```python
from build123d import *

# Parameters (mm, degrees)
SKETCH1_W               = 96
SKETCH1_H               = 64
BOSS_EXTRUDE1_DEPTH     = 20
BOSS_EXTRUDE2_DEPTH     = 32
BOSS_EXTRUDE3_DEPTH     = 12
SKETCH8_R               = 26
SKETCH8_R_2             = 16
BOSS_EXTRUDE4_DEPTH     = 32
CUT_EXTRUDE1_DEPTH      = 177.853582377
CUT_EXTRUDE1_DEPTH_BACK = 177.853582377
SKETCH9_R               = 16
RIB9_START              = -6
RIB9_DEPTH              = 12
FILLET1_R               = 1


with BuildPart() as part:
    # Sketch1 → Boss-Extrude1 (new body)
    with BuildSketch(Plane(origin=(0, 0, 0), x_dir=(1, 0, 0), z_dir=(0, 1, 0))):
        Rectangle(SKETCH1_W, SKETCH1_H)
    extrude(amount=-BOSS_EXTRUDE1_DEPTH)

    # Sketch4 → Boss-Extrude2 (add, symmetric)
    with BuildSketch(Plane(origin=(0, 0, 0), x_dir=(0, 0, -1), z_dir=(1, 0, 0))):
        with BuildLine():
            Line((20, -20), (32, -20))
            Line((32, -20), (32, 44.558859159))
            ThreePointArc((32, 44.558859159), (32.694245739, 49.069446152), (34.712719336, 53.162505705))
            Line((34.712719336, 53.162505705), (68.042689949, 100.762636801))
            Line((68.042689949, 100.762636801), (58.212865417, 107.645554037))
            Line((58.212865417, 107.645554037), (22.712719336, 56.946091171))
            ThreePointArc((22.712719336, 56.946091171), (20.694245739, 52.853031619), (20, 48.342444626))
            Line((20, 48.342444626), (20, -20))
        make_face()
    extrude(amount=BOSS_EXTRUDE2_DEPTH, both=True)

    # Sketch6 → Boss-Extrude3 (add)
    with BuildSketch(Plane(origin=(0, 8.063203075, 11.515447399), x_dir=(1, 0, 0), z_dir=(0, 0.573576436351053, 0.819152044288987))):
        with BuildLine():
            Line((-32, 121.567603544), (32, 121.567603544))
            ThreePointArc((32, 121.567603544), (0, 153.567603544), (-32, 121.567603544))
        make_face()
    extrude(amount=-BOSS_EXTRUDE3_DEPTH)

    # Sketch8 → Boss-Extrude4 (add)
    with BuildSketch(Plane(origin=(0, 8.063203075, 11.515447399), x_dir=(1, 0, 0), z_dir=(0, 0.573576436351053, 0.819152044288987))):
        with Locations(Location((0, 121.567603544, 0), (0, 0, 270))):
            Circle(SKETCH8_R)
        with Locations(Location((0, 121.567603544, 0), (0, 0, 270))):
            Circle(SKETCH8_R_2, mode=Mode.SUBTRACT)
    extrude(amount=BOSS_EXTRUDE4_DEPTH)

    # Sketch9 → Cut-Extrude1 (cut, two sides: drawn at the far end of the back side and taken through both)
    with BuildSketch(Plane(origin=(0, 8.063203075, 11.515447399), x_dir=(1, 0, 0), z_dir=(0, 0.573576436351053, 0.819152044288987)).offset(-CUT_EXTRUDE1_DEPTH_BACK)):
        with Locations(Location((0, 121.567603544, 0), (0, 0, 270))):
            Circle(SKETCH9_R)
    extrude(amount=CUT_EXTRUDE1_DEPTH + CUT_EXTRUDE1_DEPTH_BACK, mode=Mode.SUBTRACT)

    # Rib9: read off the stored shape, not the designer's step
    # Rib9 outline → Rib9 (add)
    with BuildSketch(Plane(origin=(0, 0, 0), x_dir=(0, 0, -1), z_dir=(1, 0, 0)).offset(RIB9_START)):
        with BuildLine():
            Line((22.712719336, 56.946091171), (43.702401809, 86.922464357))
            Line((43.702401809, 86.922464357), (22.404448657, 101.835451702))
            Line((22.404448657, 101.835451702), (1.414766184, 71.859078516))
            ThreePointArc((1.414766184, 71.859078516), (-4.102394981, 60.671382406), (-6, 48.342444626))
            ThreePointArc((-6, 48.342444626), (-12.91230776, 20.897080936), (-32, 0))
            Line((-32, 0), (20, 0))
            Line((20, 0), (20, 48.342444626))
            ThreePointArc((20, 48.342444626), (20.694245739, 52.853031619), (22.712719336, 56.946091171))
        make_face()
    extrude(amount=RIB9_DEPTH)

    # Fillet1
    # the kernel refuses this fillet: 1 mm, written as the material it adds along each edge
    with BuildSketch(Plane(origin=(-7, 1, -19), x_dir=(1, 0, 0), z_dir=(0, -1, 0))) as fillet1_piece_1_section:
        Polygon((0, 0), (FILLET1_R * 1.02, 0), (FILLET1_R * 1.02, -FILLET1_R * 1.02), (0, -FILLET1_R * 1.02), align=None)
    fillet1_piece_1 = extrude(amount=FILLET1_R * 1.02, mode=Mode.PRIVATE)
    fillet1_piece_1 = fillet1_piece_1 - Plane(origin=(-7, 1, -19), x_dir=(-0.7071067811865475, 0, 0.7071067811865475), z_dir=(0, -1, 0)) * Sphere(FILLET1_R, mode=Mode.PRIVATE)
    add(fillet1_piece_1)
    with BuildSketch(Plane(origin=(7, 1, -19), x_dir=(0, 0, -1), z_dir=(-1, 0, 0))) as fillet1_piece_2_section:
        Polygon((0, 0), (FILLET1_R * 1.02, 0), (FILLET1_R * 1.02, FILLET1_R * 1.02), (0, FILLET1_R * 1.02), align=None)
    fillet1_piece_2 = extrude(amount=FILLET1_R * 1.02, mode=Mode.PRIVATE)
    fillet1_piece_2 = fillet1_piece_2 - Plane(origin=(7, 1, -19), x_dir=(0, 0.7071067811865475, 0.7071067811865476), z_dir=(-1, 0, 0)) * Sphere(FILLET1_R, mode=Mode.PRIVATE)
    add(fillet1_piece_2)
    with BuildSketch(Plane(origin=(-6, 0, 34.5), x_dir=(-1, 0, 0), z_dir=(0, 0, -1))) as fillet1_piece_3_section:
        with BuildLine():
            CenterArc((FILLET1_R, FILLET1_R), FILLET1_R, 180, 90)
            Line((0, FILLET1_R), (0, 0))
            Line((0, 0), (FILLET1_R, 0))
        make_face()
    fillet1_piece_3 = extrude(amount=53.5, mode=Mode.PRIVATE)
    fillet1_piece_3 = fillet1_piece_3 - Plane(origin=(-6, 48.342444627, 63.942152933), x_dir=(0, -1.6764948068756696e-11, -1.0), z_dir=(-1, 0, 0)) * Cylinder(57.942152933, 111, mode=Mode.PRIVATE)
    add(fillet1_piece_3)
    with BuildSketch(Plane(origin=(-6, 1, -20), x_dir=(0, 0, 1), z_dir=(0, 1, 0)), Plane(origin=(6, 1, -20), x_dir=(1, 0, 0), z_dir=(0, 1, 0))) as fillet1_piece_4:
        with BuildLine():
            CenterArc((FILLET1_R, -FILLET1_R), FILLET1_R, 90, 90)
            Line((0, -FILLET1_R), (0, 0))
            Line((0, 0), (FILLET1_R, 0))
        make_face()
    extrude(amount=47.342444626)
    with BuildSketch(Plane(origin=(-6, 48.342444626, -34.999999997), x_dir=(0, -1.1790272464341429e-11, 1.0), z_dir=(0, -1.0, -1.1790272464341429e-11))) as fillet1_piece_5:
        with BuildLine():
            CenterArc((14.999999997 + FILLET1_R, FILLET1_R), FILLET1_R, 180, 90)
            Line((14.999999997, FILLET1_R), (14.999999997, 0))
            Line((14.999999997, 0), (14.999999997 + FILLET1_R, 0))
        make_face()
    revolve(axis=Axis((-6, 48.342444626, -34.999999997), (-1, 0, 0)), revolution_arc=35.000000006)
    with BuildSketch(Plane(origin=(-6, 56.946091171, -22.712719336), x_dir=(0, 0.5735764363505949, 0.8191520442893078), z_dir=(0, 0.8191520442893078, -0.5735764363505949))) as fillet1_piece_6:
        with BuildLine():
            CenterArc((FILLET1_R, -FILLET1_R), FILLET1_R, 90, 90)
            Line((FILLET1_R * 4.36944609845e-10, -FILLET1_R), (0, 0))
            Line((0, 0), (FILLET1_R, 0))
        make_face()
    extrude(amount=39.09439465)
    with BuildSketch(Plane(origin=(-7, 0, -20), x_dir=(0, 0, 1), z_dir=(-1, 0, 0)), Plane(origin=(32, 0, -20), x_dir=(0, 0, 1), z_dir=(-1, 0, 0))) as fillet1_piece_7:
        with BuildLine():
            CenterArc((FILLET1_R, FILLET1_R), FILLET1_R, 180, 90)
            Line((0, FILLET1_R), (0, 0))
            Line((0, 0), (FILLET1_R, 0))
        make_face()
    extrude(amount=25)
    with BuildSketch(Plane(origin=(0, 107.645554037, -58.212865417), x_dir=(0.13576209912183695, -0.8115678972317177, 0.5682659594106623), z_dir=(-0.990741465995056, -0.11120980103261684, 0.07786994100584167))) as fillet1_piece_8:
        with BuildLine():
            CenterArc((26 + FILLET1_R, FILLET1_R), FILLET1_R, 180, 90)
            Line((26, FILLET1_R), (26, 0))
            Line((26, 0), (26 + FILLET1_R, 0))
        make_face()
    revolve(axis=Axis((0, 107.645554037, -58.212865417), (0, 0.573576436351053, 0.819152044288987)), revolution_arc=344.394618628)
    with BuildSketch(Plane(origin=(6, 0, 34.5), x_dir=(1, 0, 0), z_dir=(0, 0, -1))) as fillet1_piece_9_section:
        with BuildLine():
            CenterArc((FILLET1_R, -FILLET1_R), FILLET1_R, 90, 90)
            Line((0, -FILLET1_R), (0, 0))
            Line((0, 0), (FILLET1_R, 0))
        make_face()
    fillet1_piece_9 = extrude(amount=53.5, mode=Mode.PRIVATE)
    fillet1_piece_9 = fillet1_piece_9 - Plane(origin=(6, 48.342444627, 63.942152933), x_dir=(0, -1.6764948068756696e-11, -1.0), z_dir=(-1, 0, 0)) * Cylinder(57.942152933, 111, mode=Mode.PRIVATE)
    add(fillet1_piece_9)
    with BuildSketch(Plane(origin=(6, 48.342444626, -34.999999997), x_dir=(0, -1.1790272464341429e-11, 1.0), z_dir=(0, -1.0, -1.1790272464341429e-11))) as fillet1_piece_10:
        with BuildLine():
            CenterArc((14.999999997 + FILLET1_R, -FILLET1_R), FILLET1_R, 90, 90)
            Line((14.999999997, -FILLET1_R), (14.999999997, 0))
            Line((14.999999997, 0), (14.999999997 + FILLET1_R, 0))
        make_face()
    revolve(axis=Axis((6, 48.342444626, -34.999999997), (-1, 0, 0)), revolution_arc=35.000000006)
    with BuildSketch(Plane(origin=(6, 56.946091171, -22.712719336), x_dir=(0, 0.5735764363505949, 0.8191520442893078), z_dir=(0, 0.8191520442893078, -0.5735764363505949))) as fillet1_piece_11:
        with BuildLine():
            CenterArc((FILLET1_R, FILLET1_R), FILLET1_R, 180, 90)
            Line((FILLET1_R * 4.36944609845e-10, FILLET1_R), (0, 0))
            Line((0, 0), (FILLET1_R, 0))
        make_face()
    extrude(amount=39.09439465)


solid = part.part
```
Input: part model. Units: mm. Frame: model coordinates. A direction names the side the tool comes from. Give positions to 0.01 mm unless a question says otherwise; leave off trailing zeros. Order: outer loops, then holes, each group sorted by start corner. A loop starts at its lowest first (then second) coordinate and runs counter-clockwise, first axis right, second up.
1. Cut plane B-B (z = 3). Return loops of the section in (x, y).
Computed:
outline: (-48, -20) - (48, -20) - (48, 0) - (7, 0) arc R1 cw to (6, 1) - (6, 63.74) - (-6, 63.74) - (-6, 1) arc R1 cw to (-7, 0) - (-48, 0) - close
2. Line query: probe 1 along Y at (x, z) = (-42, 9.5); probe 2 along X at (y, z) = (55, -16.5); probe 3 along X at (y, z) = (109, -43). Output: solid intervals per line, ascending.
Computed:
probe 1: y = -20 to 0
probe 2: x = -6 to 6
probe 3: x = -24.86 to -14.07, 14.07 to 24.86
3. Draft query along Y for faces 6 (the face through (-19.325, 52.914, -20.714)), 7 (the face through (-0.08, 60.84, 4.05)), 8 (the face through (-1, 13, -32)). Return one class per face: released by +Y, released by -Y, zero draft, split by the parting line, or undercut.
Computed:
face 6: undercut
face 7: released by +Y
face 8: zero draft
4. Cut plane C-C (x = -34). Return loops of the section in (y, z).
Computed:
outline: (-20, -32) - (0, -32) - (0, 32) - (-20, 32) - close
5. Set-up query: faces 1 (the face through (20, 25, -20)), 2 (the face through (-6, 52, -6)), 3 (the face through (-32, 54, -34)), 4 (the face through (-1, -10, 32)), 5 (the face through (-48, -10, 0)). Return all of +Z, -Z, +X, -X, +Y, -Y with unobstructed straight access to the full face (end or side cutting, diameter ignored); none if empty.
Computed:
face 1: +Z, +X
face 2: +Z, -X
face 3: +Z, -Z, -X, +Y
face 4: +Z, +X, -X, +Y, -Y
face 5: +Z, -Z, -X, +Y, -Y
6. Pin query (flat end, axial travel): pin 1 Ø2 at (x, y) = (17, 35) entering from +Z; pin 2 Ø1.5 at (x, z) = (-34.5, -42.5) entering from -Y; pin 3 Ø6 at (y, z) = (25.5, -2.5) entering from -X; pin 4 Ø24.5 at (y, z) = (74, -44) entering from -X. Return the tip coordinate at first contact, or that it passes through.
Computed:
pin 1: stops at z = -20
pin 2: passes through
pin 3: stops at x = -6
pin 4: stops at x = -32
7. Cut plane A-A (y = 27.5). Return loops of the section in (x, z), and give its area (3 significant figures).
Computed:
outline: (-32, -32) - (32, -32) - (32, -20) - (7, -20) arc R1 cw to (6, -19) - (6, 9.88) - (-6, 9.88) - (-6, -19) arc R1 cw to (-7, -20) - (-32, -20) - close
area: 1,130 mm2
